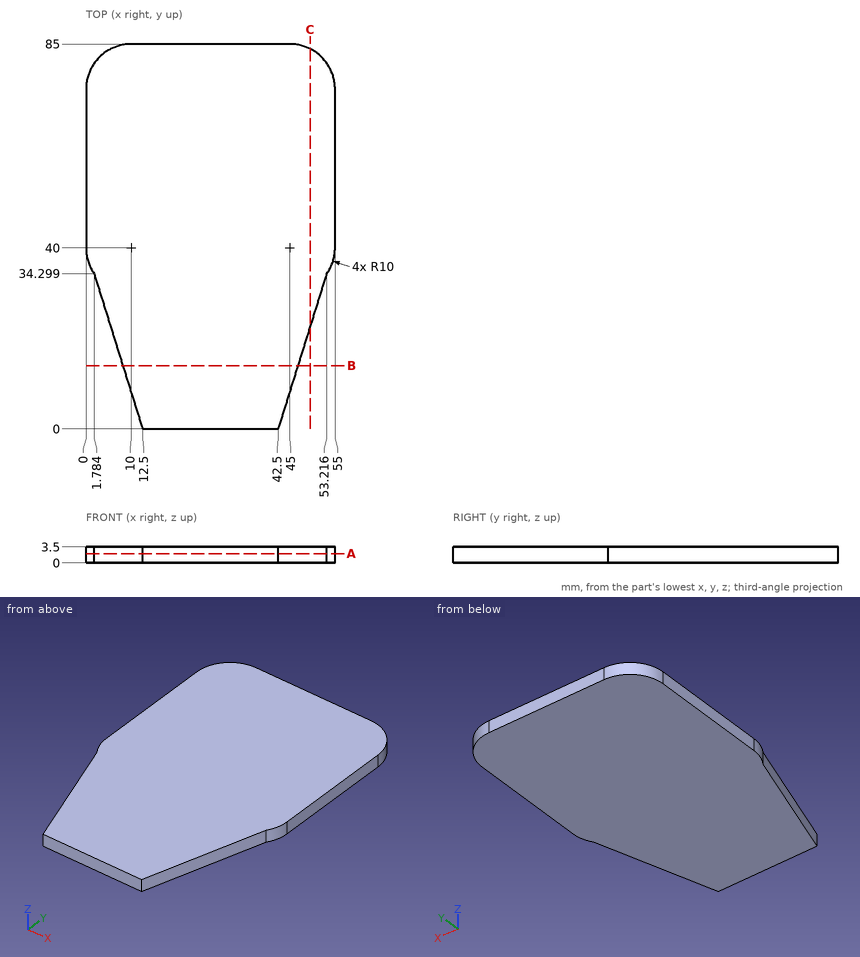
Here's the drawing with two shaded views (mm, measured from the low corner). I have some questions. Give positions to 0.01 mm unless a question says otherwise; leave off trailing zeros. Loops run counter-clockwise (first coordinate to the right, second up) from the corner with the lowest first, then second, coordinate; pieces in that order, holes last. Notation, with made-up numbers: (42.25, -0.5) - (59.25, -0.5) arc R25 ccw to (59.25, 12.5) - close; hole circle Ø5 at (-34.5, 38.5). An arc over 180 degrees is marked (long way). Answer in a Markdown table with one row per item. Add a question column.
Q1. If we section it at B-B (y = 14): List the corners of the cut face in (x, z) for me.
Q2. If we section it at C-C (x = 49.5): List the corners of the cut face in (y, z) for me.
Q3. If we section it at A-A (z = 2): List the corners of the cut face in (x, y) for me.
Q4. Please list where these lines run through material, in increasing order: L1, parallel to X at y = 81, z = 2; L2, parallel to X at y = 78, z = 1.65. Write a range as from..to.
The answers:
| question | item | result |
|---|---|---|
| 1 | outline | (8.13, 0) - (46.87, 0) - (46.87, 3.5) - (8.13, 3.5) - close |
| 2 | outline | (22.41, 0) - (83.93, 0) - (83.93, 3.5) - (22.41, 3.5) - close |
| 3 | outline | (0, 40) arc R10 ccw to (1.78, 34.3) - (12.5, 0) - (42.5, 0) - (53.22, 34.3) arc R10 ccw to (55, 40) - (55, 75) arc R10 ccw to (45, 85) - (10, 85) arc R10 ccw to (0, 75) - close |
| 4 | L1 | x = 2..53 |
| 4 | L2 | x = 0.46..54.54 |
